```python
from build123d import *

# Parameters (mm, degrees)
BOSS_EXTRUDE1_DEPTH = 3
BOSS_EXTRUDE2_START = -1.75
BOSS_EXTRUDE2_DEPTH = 1.75
SKETCH2_R           = 1.75
CUT_EXTRUDE1_DEPTH  = 4.75
SKETCH2_3_R         = 3
CUT_EXTRUDE2_DEPTH  = 1.75
SKETCH1_6_W         = 11
SKETCH1_6_H         = 6
BOSS_EXTRUDE3_DEPTH = 5
SKETCH3_R           = 1.35
CUT_EXTRUDE3_DEPTH  = 8
LPATTERN1_COUNT     = 2
LPATTERN1_PITCH     = 8
LPATTERN1_COL_COUNT = 2
LPATTERN1_COL_PITCH = 8


with BuildPart() as part:
    # Sketch1 → Boss-Extrude1 (new body)
    with BuildSketch(Plane.XY):
        with BuildLine():
            Line((-11, 30), (-11, -30))
            Line((-11, -30), (11, -30))
            Line((11, -30), (11, 30))
            ThreePointArc((11, 30), (0, 41), (-11, 30))
        make_face()
        with BuildLine():
            Line((5, -23), (-5, -23))
            Line((-5, -23), (-5, 19.643842411))
            ThreePointArc((-5, 19.643842411), (0, 18.5), (5, 19.643842411))
            Line((5, 19.643842411), (5, -23))
        make_face(mode=Mode.SUBTRACT)
    extrude(amount=BOSS_EXTRUDE1_DEPTH)

    # Sketch1<3> → Boss-Extrude2 (add)
    with BuildSketch(Plane.XY.offset(BOSS_EXTRUDE2_START)):
        with BuildLine():
            ThreePointArc((11, 30), (0, 41), (-11, 30))
            ThreePointArc((-11, 30), (0, 19), (11, 30))
        make_face()
    extrude(amount=BOSS_EXTRUDE2_DEPTH)

    # Sketch2 → Cut-Extrude1 (cut)
    with BuildSketch(Plane.XY.offset(3)):
        with Locations((0, 30)):
            Circle(SKETCH2_R)
    extrude(amount=-CUT_EXTRUDE1_DEPTH, mode=Mode.SUBTRACT)

    # Sketch2<3> → Cut-Extrude2 (cut)
    with BuildSketch(Plane.XY.offset(3)):
        with Locations((0, 30)):
            Circle(SKETCH2_3_R)
    extrude(amount=-CUT_EXTRUDE2_DEPTH, mode=Mode.SUBTRACT)

    # Sketch1<6> → Boss-Extrude3 (add)
    with BuildSketch(Plane.XY):
        with Locations((5.5, -27)):
            Rectangle(SKETCH1_6_W, SKETCH1_6_H)
        with Locations((-5.5, -27)):
            Rectangle(SKETCH1_6_W, SKETCH1_6_H)
    extrude(amount=-BOSS_EXTRUDE3_DEPTH)

    # Sketch3 → Cut-Extrude3 (cut)
    with BuildSketch(Plane.XY.offset(3)):
        with Locations((0, -26.6)):
            Circle(SKETCH3_R)
    cut_extrude3 = extrude(amount=-CUT_EXTRUDE3_DEPTH, mode=Mode.SUBTRACT)

    # LPattern1: Cut-Extrude3 ×2
    with Locations(*[(i * LPATTERN1_PITCH, 0, 0) for i in range(1, LPATTERN1_COUNT)]):
        add(cut_extrude3, mode=Mode.SUBTRACT)

    # LPattern1 col: Cut-Extrude3 ×2
    with Locations(*[(-i * LPATTERN1_COL_PITCH, 0, 0) for i in range(1, LPATTERN1_COL_COUNT)]):
        add(cut_extrude3, mode=Mode.SUBTRACT)


solid = part.part
```
Design review of the part built by this model. Coordinates are the model's own, in mm. A direction names the side the tool comes from. Coordinates: 2 decimals unless noted, no trailing zeros. Loops run counter-clockwise (first coordinate to the right, second up) from the corner with the lowest first, then second, coordinate; pieces in that order, holes last. Notation, with made-up numbers: M 6.25,-13.75 L 21.25,-13.75 A20 cw 21.25,13.25 Z; hole C 20.5,-6.75 d5. An arc over 180 degrees is marked long. One line per question, with ' | ' between items.
(1) For pin 1 Ø5.5 at (x, y) = (0, 30) entering from +Z; pin 2 Ø6.5 at (x, y) = (2.5, -8.5) entering from -Z; pin 3 Ø5.5 at (x, y) = (0, 30) entering from -Z, all flat-tipped, find the tip position at first contact; note any pin that passes through.
Filled in:
pin 1: stops at z = 1.25 | pin 2: stops at z = 0 | pin 3: stops at z = -1.75
(2) Draft analysis for pull direction Y (two halves, no side actions). For faces 5 (the face through (0, -30, -1)), 6 (the face through (-0.2, -28.3, -5)), 7 (the face through (0, -23, 1)), state which applies: released by +Y, released by -Y, zero draft, split by the parting line, or undercut.
Filled in:
face 5: released by -Y | face 6: zero draft | face 7: undercut
(3) We need section B-B (y = -4). Give the boundary of the cut face in (x, z).
Filled in:
outline: M -11,0 L -5,0 L -5,3 L -11,3 Z; M 5,0 L 11,0 L 11,3 L 5,3 Z
(4) Wall thickness on probe 1 along Y at (x, z) = (0, 0.25); probe 2 along Y at (x, z) = (0, -0.85); probe 3 along X at (y, z) = (5, 1): over which ranges is each line inside the solid? List them lowest first.
Filled in:
probe 1: y = -30 to -27.95, -25.25 to -23, 18.5 to 28.25, 31.75 to 41 | probe 2: y = -30 to -27.95, -25.25 to -24, 19 to 28.25, 31.75 to 41 | probe 3: x = -11 to -5, 5 to 11
(5) We need section D-D (x = 0). Give the boundary of the cut face in (y, z).
Filled in:
outline: M -30,-5 L -27.95,-5 L -27.95,3 L -30,3 Z; M -25.25,-5 L -24,-5 L -24,0 L -23,0 L -23,3 L -25.25,3 Z; M 18.5,0 L 19,0 L 19,-1.75 L 28.25,-1.75 L 28.25,1.25 L 27,1.25 L 27,3 L 18.5,3 Z; M 31.75,-1.75 L 41,-1.75 L 41,3 L 33,3 L 33,1.25 L 31.75,1.25 Z
(6) We need section A-A (y = -26.6). Give the boundary of the cut face in (x, z).
Filled in:
outline: M -11,-5 L -9.35,-5 L -9.35,3 L -11,3 Z; M -6.65,-5 L -1.35,-5 L -1.35,3 L -6.65,3 Z; M 1.35,-5 L 6.65,-5 L 6.65,3 L 1.35,3 Z; M 9.35,-5 L 11,-5 L 11,3 L 9.35,3 Z
(7) Machinability: for faces 1 (the face through (5, -1, 1)), 2 (the face through (2.38, 40.74, 0.06)), 3 (the face through (0, 28, -1.75)), 4 (the face through (0, 28, 1.25)), which of the approach directions +Z, -Z, +X, -X, +Y, -Y give a long, thin tool a straight path to every point of the face, cutting with its end or side? Answer none if there is none.
Filled in:
face 1: +Z, -Z | face 2: -Z | face 3: -Z, +X, -X, +Y | face 4: +Z
(8) We need section C-C (z = -2.5). Give the boundary of the cut face in (x, y), and give its area (3 significant figures).
Filled in:
outline: M -11,-30 L 11,-30 L 11,-24 L -11,-24 Z; hole C -8,-26.6 d2.7; hole C 0,-26.6 d2.7; hole C 8,-26.6 d2.7 | area: 115 mm^2
